from build123d import *

# Parameters (mm, degrees)
F0_W     = 381
F0_H     = 260.35
F1_DEPTH = 19.05
F2_SIZE  = 19.04999


# Not quite as in the source:
# - a fillet or chamfer is up to 0.001 mm smaller than in the source, because OpenCascade refuses the exact size


with BuildPart() as f1:
    # F0 (on Right) → F1 (new body)
    with BuildSketch(Plane.YZ):
        Rectangle(F0_W, F0_H)
    extrude(amount=F1_DEPTH)

    # F2 (size 19.05 in the source; OpenCascade refuses exactly that, so slightly less here)
    f2_edges = [f1.edges().sort_by_distance(p)[0] for p in [
        (0, 0, -130.175),
        (0, 0, 130.175),
        (0, -190.5, 0),
    ]]
    chamfer(f2_edges, length=F2_SIZE)


solid = f1.part
Geometry: final body of the model. Coordinates: model frame, mm. Coordinates: 2 decimals unless noted, no trailing zeros. Order: outer loops, then holes, each group sorted by start corner. A loop starts at its lowest first (then second) coordinate and runs counter-clockwise, first axis right, second up. Notation, with made-up numbers: M 3.25,-38.5 L 38.25,-38.5 A24 ccw 38.25,-1.5 Z; hole C 15,70 d11. An arc over 180 degrees is marked long. One line per question, with ' | ' between items. Start each with the question number.
Item 1: Pin query (flat end, axial travel): pin 1 Ø1 at (x, z) = (6, -1.5) entering from -Y; pin 2 Ø5 at (x, y) = (13, 125) entering from -Z (3 decimals); pin 3 Ø2 at (x, y) = (10, 5.5) entering from -Z (3 decimals). Return the tip coordinate at first contact, or that it passes through.
Item 2: Ray query, probe 1 along Z at (x, y) = (18.25, 173.5); probe 2 along Z at (x, y) = (6.75, -161); probe 3 along Y at (x, z) = (6.25, -42). Return the intervals inside material, ascending. Write a range as [from, to].
Item 3: Cut plane C-C, the plane x = 16. Return the cut outline in (y, z) (3 decimals).
A:
1) pin 1: stops at y = -177.95 | pin 2: stops at z = -126.625 | pin 3: stops at z = -122.125
2) probe 1: z = [-129.38, 129.38] | probe 2: z = [-117.88, 117.88] | probe 3: y = [-177.7, 190.5]
3) outline: M -187.45,-127.125 L 190.5,-127.125 L 190.5,127.125 L -187.45,127.125 Z
